```python
from build123d import *

# Parameters (mm, degrees)
REVOLU_O2_ANGLE          = 50
RESSALTO_EXTRUS_O1_START = -100
RESSALTO_EXTRUS_O1_DEPTH = 100
ESBO_O9_W                = 82
ESBO_O9_H                = 36
CORTE_EXTRUS_O6_DEPTH    = 147.5
ESBO_O11_W               = 72
ESBO_O11_H               = 25
CORTE_EXTRUS_O7_DEPTH    = 172
ESBO_O15_R               = 3.5
CORTE_EXTRUS_O8_DEPTH    = 49
ESBO_O16_W               = 86
ESBO_O16_H               = 40
ESBO_O16_W_2             = 82
ESBO_O16_H_2             = 36
CORTE_EXTRUS_O9_DEPTH    = 135
ESBO_O17_W               = 9.4
ESBO_O17_H               = 35.4
CORTE_EXTRUS_O10_DEPTH   = 30
ESBO_O18_R               = 3
CORTE_EXTRUS_O12_DEPTH   = 5
FILETE1_R                = 10


with BuildPart() as part:
    # Esboço1 → Revolução2 (revolve, symmetric)
    with BuildSketch(Plane.XY) as revolu_o2_sk:
        Polygon((133.047501561, 1), (132.06191984, -18.71163442), (117.080634756, -17.962570166), (118.578763265, 12), (150.6, 12), (150.6, -88), (130.6, -88), (135.05, 1), align=None)
    revolve(axis=Axis((0, -200, 0), (0, 1, 0)), revolution_arc=REVOLU_O2_ANGLE / 2)
    revolve(revolu_o2_sk.sketch, axis=Axis((0, -200, 0), (0, -1, 0)), revolution_arc=REVOLU_O2_ANGLE / 2)

    # Esboço10 → Ressalto-extrusão1 (add)
    with BuildSketch(Plane(origin=(0, 12, 0), x_dir=(1, 0, 0), z_dir=(0, 1, 0)).offset(RESSALTO_EXTRUS_O1_START)):
        with BuildLine():
            Line((152.489952728, 0), (150.6, 0))
            ThreePointArc((150.6, 0), (147.030178672, -32.595805859), (136.489952728, -63.646310218))
            Line((136.489952728, -63.646310218), (152.489952728, -50))
            Line((152.489952728, -50), (152.489952728, 0))
        make_face()
        with BuildLine():
            Line((152.489952728, 50), (136.489952728, 63.646310218))
            ThreePointArc((136.489952728, 63.646310218), (147.030178672, 32.595805859), (150.6, 0))
            Line((150.6, 0), (152.489952728, 0))
            Line((152.489952728, 0), (152.489952728, 50))
        make_face()
    extrude(amount=RESSALTO_EXTRUS_O1_DEPTH)

    # Esboço9 → Corte-extrusão6 (cut)
    with BuildSketch(Plane(origin=(0, 0, 0), x_dir=(0, 0, -1), z_dir=(1, 0, 0))):
        with Locations((0, -55)):
            Rectangle(ESBO_O9_W, ESBO_O9_H)
    extrude(amount=CORTE_EXTRUS_O6_DEPTH, mode=Mode.SUBTRACT)

    # Esboço11 → Corte-extrusão7 (cut)
    with BuildSketch(Plane(origin=(0, 0, 0), x_dir=(0, 0, -1), z_dir=(1, 0, 0))):
        with Locations((0, -55)):
            Rectangle(ESBO_O11_W, ESBO_O11_H)
    extrude(amount=CORTE_EXTRUS_O7_DEPTH, mode=Mode.SUBTRACT)

    # Esboço15 → Corte-extrusão8 (cut)
    with BuildSketch(Plane(origin=(0, 12, 0), x_dir=(1, 0, 0), z_dir=(0, 1, 0))):
        with Locations(Location((138.649952728, -30, 0), (0, 0, 270))):
            Circle(ESBO_O15_R)
    extrude(amount=-CORTE_EXTRUS_O8_DEPTH, mode=Mode.SUBTRACT)

    # Esboço16 → Corte-extrusão9 (cut)
    with BuildSketch(Plane(origin=(0, 0, 0), x_dir=(0, 0, -1), z_dir=(1, 0, 0))):
        with Locations((0, -55)):
            Rectangle(ESBO_O16_W, ESBO_O16_H)
        with Locations((0, -55)):
            Rectangle(ESBO_O16_W_2, ESBO_O16_H_2, mode=Mode.SUBTRACT)
    extrude(amount=CORTE_EXTRUS_O9_DEPTH, mode=Mode.SUBTRACT)

    # Esboço17 → Corte-extrusão10 (cut)
    with BuildSketch(Plane(origin=(0, 12, 0), x_dir=(1, 0, 0), z_dir=(0, 1, 0))):
        with Locations((142.789952728, 0)):
            Rectangle(ESBO_O17_W, ESBO_O17_H)
    extrude(amount=-CORTE_EXTRUS_O10_DEPTH, mode=Mode.SUBTRACT)

    # Esboço18 → Corte-extrusão12 (cut)
    with BuildSketch(Plane(origin=(152.489952728, 0, 0), x_dir=(0, 0, -1), z_dir=(1, 0, 0))):
        with Locations((0, 4.465209406)):
            Circle(ESBO_O18_R)
    extrude(amount=-CORTE_EXTRUS_O12_DEPTH, mode=Mode.SUBTRACT)

    # Filete1
    filete1_edges = [part.edges().sort_by_distance(p)[0] for p in [
        (117.080634756, -17.962570166, 0),
        (152.489952728, -38, -50),
        (152.489952728, -38, 50),
        (136.489952728, -38, -63.646310218),
        (136.489952728, -38, 63.646310218),
    ]]
    fillet(filete1_edges, radius=FILETE1_R)


solid = part.part
```
Check sheet for the modelled part. Datum: model origin and axes. Units: mm. A direction names the side the tool comes from. Round coordinates to 2 decimals unless told otherwise and drop trailing zeros. Loops run counter-clockwise (first coordinate to the right, second up) from the corner with the lowest first, then second, coordinate; pieces in that order, holes last. Notation, with made-up numbers: (-26, 24.5) - (29, 24.5) arc R18 cw to (29, 48.5) - close; hole circle Ø10 at (-30.75, 25). An arc over 180 degrees is marked (long way). Answer as a JSON object with one key per item and string values. Group by question number.
Q1. Sectioned sample at B-B, the plane y = -24. Enter the section's corners in (x, z), plus the area to 3 significant figures.
Q2. Set-up check for faces 1 (the face through (150, -67.5, 1)), 2 (the face through (147.5, -68, 3)), 3 (the face through (143, -3, 17.7)), 4 (the face through (134, 1, 0)): record each of +Z, -Z, +X, -X, +Y, -Y from which the full face is reachable in a straight line by a thin tool's end or side.
Q3. Sectioned sample at C-C, the plane x = 144. Enter the section's corners in (y, z), plus the area to 3 significant figures.
Q4. Sectioned sample at D-D, the plane z = 30. Count the separate pieces of the cut face and the enclosed holes in it, plus the area to 3 significant figures.
Q5. Mould release check, pull along Z, two halves, no side actions. Record for faces 5 (the face through (145.23, -38.7, -56.19)), 6 (the face through (129, -55, -43)), 7 (the face through (152.49, -39, 1)): released by +Z, released by -Z, zero draft, split by the parting line, or undercut.
Q6. Scan lines: line 1 along Y through (x, z) = (150, 0); line 2 along X through (y, z) = (-2, 10.5); line 3 along Z through (x, y) = (140, -12). Record each from-to range of solid material in increasing order. Write a range as [from, to].
Q7. Gauge pin test, flat ends, axial feed: P1, Ø10, axis at x = 112, z = 43.5, coming from the -Y side; P2, Ø5.5, axis at x = 127, y = -55, coming from the -Z side; P3, Ø2.5, axis at x = 150.5, y = -57, coming from the +Z side; P4, Ø2, axis at x = 147, z = 1.5, coming from the +Y side. Record the tip position at first contact, or that the pin passes through.
Q8. Sectioned sample at A-A, the plane y = -58. Enter the section's corners in (x, z), plus the area to 3 significant figures.
Solution:
{
 "1": {"outline": "(121.26, -56.55) - (130.66, -60.93) arc R10 ccw to (141.38, -59.48) - (148.98, -52.99) arc R10 ccw to (152.49, -45.39) - (152.49, 45.39) arc R10 ccw to (148.98, 52.99) - (141.38, 59.48) arc R10 ccw to (130.66, 60.93) - (121.26, 56.55) arc R133.8 cw to start; hole circle Ø7 at (138.65, 30)", "area": "2,640 mm²"},
 "2": {"face 1": "+X, -X", "face 2": "-X", "face 3": "+Y", "face 4": "none"},
 "3": {"outline": "(-88, -57.24) - (12, -57.24) - (12, -17.7) - (-18, -17.7) - (-18, 17.7) - (12, 17.7) - (12, 57.24) - (-88, 57.24) - close; hole (-73, -41) - (-37, -41) - (-37, 41) - (-73, 41) - close", "area": "7,430 mm²"},
 "4": {"separate pieces": "3", "enclosed holes": "0", "area": "1,590 mm²"},
 "5": {"face 5": "released by -Z", "face 6": "undercut", "face 7": "zero draft"},
 "6": {"line 1": "y = [-88, -67.5], [-42.5, 1.47], [7.47, 12]", "line 2": "x = [117.41, 132.48], [134.49, 138.09], [147.49, 152.49]", "line 3": "z = [-60.46, -17.7], [17.7, 26.77], [33.23, 60.46]"},
 "7": {"P1": "stops at y = -18.18", "P2": "stops at z = -60.5", "P3": "stops at z = 52.75", "P4": "stops at y = 12"},
 "8": {"outline": "(119.72, -55.83) - (130.66, -60.93) arc R10 ccw to (141.38, -59.48) - (148.98, -52.99) arc R10 ccw to (152.49, -45.39) - (152.49, -36) - (147.5, -36) - (147.5, -41) - (135, -41) - (135, -43) - (124.91, -43) arc R132.1 cw to start; (119.72, 55.83) arc R132.1 cw to (124.91, 43) - (135, 43) - (135, 41) - (147.5, 41) - (147.5, 36) - (152.49, 36) - (152.49, 45.39) arc R10 ccw to (148.98, 52.99) - (141.38, 59.48) arc R10 ccw to (130.66, 60.93) - close", "area": "1,030 mm²"}
}
